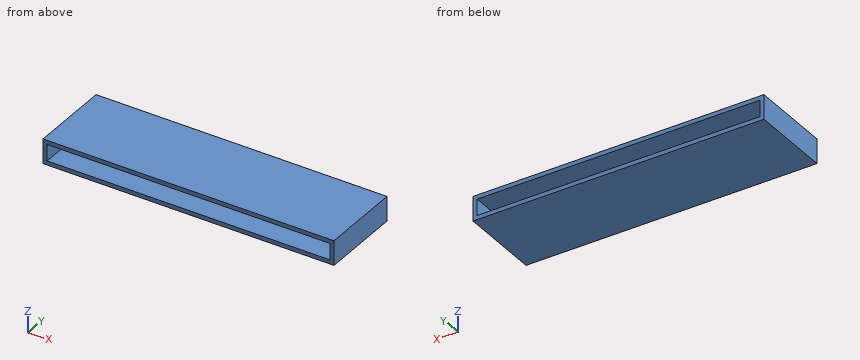
```python
from build123d import *

# Parameters (mm, degrees)
F0_W          = 2.54
F0_H          = 2.54
F3_W          = 2.54
F3_H          = 2.54
F8_DEPTH      = 25.4
F8_DEPTH_BACK = 25.4


with BuildPart() as f2:
    # F2: sweep along a path in F1
    with BuildLine(Plane.XZ) as f2_path:
        Line((118.0932859957, 0), (-59.7067140043, 0))
        Line((-59.7067140043, 0), (-59.7067140043, 12.7))
        Line((-59.7067140043, 12.7), (118.0932859957, 12.7))
        Line((118.0932859957, 12.7), (118.0932859957, 0))
    # F0 (on Right) → F2 (sweep)
    with BuildSketch(Plane.YZ):
        Rectangle(F0_W, F0_H)
    sweep(path=f2_path.line, transition=Transition.RIGHT)

    # F8 (add, two sides): a face of the model
    f8_faces = [f2.faces().sort_by_distance(p)[0] for p in [
        (29.1932859957, -1.27, 13.2398279808),
    ]]
    extrude(f8_faces, amount=F8_DEPTH)
    extrude(f8_faces, amount=-F8_DEPTH_BACK)


with BuildPart() as f6:
    # F6: sweep along a path in F5
    with BuildLine(Plane(origin=(0, 1.27, 0), x_dir=(-1, 0, 0), z_dir=(0, 1, 0))) as f6_path:
        Line((59.1895133257, 0), (-31.8534299731, 14.0118226409))
        Line((-31.8534299731, 14.0118226409), (-116.2539571524, 0))
    # F3 (on face) → F6 (sweep)
    with BuildSketch(Plane.XY.offset(13.97)):
        with Locations((31.7332859957, 0)):
            Rectangle(F3_W, F3_H)
    sweep(path=f6_path.line, transition=Transition.RIGHT)


solid = f2.part
```
Geometry: final body of the model. Coordinates: model frame, mm. Coordinates: 2 decimals unless noted, no trailing zeros. Write each loop counter-clockwise with the first axis right and the second up, starting at its lowest first coordinate (ties: lowest second). Pieces come first, ordered by that corner, then holes. Notation, with made-up numbers: M 61.25,52.5 L 114.25,52.5 A20 ccw 114.25,58.5 Z; hole C 52.25,43 d8. An arc over 180 degrees is marked long. Answer as CSV lines item,"result". Start each with the question number.
Q1. Cut plane A-A on y = -4. Return the cut outline in (x, z).
Q2. Cut plane B-B on x = -18. Return the cut outline in (y, z), then the cut area to 3 significant figures.
Q3. Line query: line 1 (Z direction, x = -20.5, y = 16); line 2 (X direction, y = 1.5, z = 6.5). Output: solid intervals per line, ascending. Write a range as from..to.
Q4. Cut plane C-C on z = 6.75. Return the cut outline in (x, y).
Q5. Pin query (flat end, axial travel): P1, Ø4, axis at x = 69.5, z = 9, coming from the +Y side. Return the tip coordinate at first contact, or that it passes through.
Findings below:
1,outline,"M -60.98,-1.27 L 119.36,-1.27 L 119.36,13.97 L -60.98,13.97 Z; hole M -58.44,1.27 L 116.82,1.27 L 116.82,11.43 L -58.44,11.43 Z"
2,outline,"M -26.67,-1.27 L 24.13,-1.27 L 24.13,1.27 L -26.67,1.27 Z; M -26.67,11.43 L 24.13,11.43 L 24.13,13.97 L -26.67,13.97 Z"
2,area,"258 mm2"
3,line 1,"z = -1.27..1.27, 11.43..13.97"
3,line 2,"x = -60.98..-58.44, 116.82..119.36"
4,outline,"M -60.98,-26.67 L -58.44,-26.67 L -58.44,24.13 L -60.98,24.13 Z; M 116.82,-26.67 L 119.36,-26.67 L 119.36,24.13 L 116.82,24.13 Z"
5,P1,"passes through"
